from build123d import *

# Parameters (mm, degrees)
SKETCH3_R           = 57.15
BOSS_EXTRUDE2_DEPTH = 6.35
SKETCH4_R           = 3.81
SKETCH4_R_2         = 12.7
CUT_EXTRUDE1_DEPTH  = 6.35
SKETCH5_R           = 1.9685
CUT_EXTRUDE2_DEPTH  = 6.35


with BuildPart() as part:
    # Sketch3 → Boss-Extrude2 (new body)
    with BuildSketch(Plane.XY):
        Circle(SKETCH3_R)
    extrude(amount=BOSS_EXTRUDE2_DEPTH)

    # Sketch4 → Cut-Extrude1 (cut)
    with BuildSketch(Plane(origin=(0, 0, 0), x_dir=(-1, 0, 0), z_dir=(0, 0, -1))):
        with Locations((-35.921024484, 35.921024484)):
            Circle(SKETCH4_R)
        with Locations((35.921024484, 35.921024484)):
            Circle(SKETCH4_R)
        with Locations((35.921024484, -35.921024484)):
            Circle(SKETCH4_R)
        with Locations((-35.921024484, -35.921024484)):
            Circle(SKETCH4_R)
        Circle(SKETCH4_R_2)
    extrude(amount=-CUT_EXTRUDE1_DEPTH, mode=Mode.SUBTRACT)

    # Sketch5 → Cut-Extrude2 (cut)
    with BuildSketch(Plane.XY.offset(6.35)):
        with Locations((-22.225, 22.225)):
            Circle(SKETCH5_R)
        with Locations((22.225, 22.225)):
            Circle(SKETCH5_R)
        with Locations((22.225, -22.225)):
            Circle(SKETCH5_R)
        with Locations((-22.225, -22.225)):
            Circle(SKETCH5_R)
    extrude(amount=-CUT_EXTRUDE2_DEPTH, mode=Mode.SUBTRACT)


solid = part.part
The listing builds one solid part. Answer for the finished solid, in the listing's coordinates (mm). Coordinates: 2 decimals unless noted, no trailing zeros. Write each loop counter-clockwise with the first axis right and the second up, starting at its lowest first coordinate (ties: lowest second). Pieces come first, ordered by that corner, then holes. Notation, with made-up numbers: M -1,-40 L 43,-40 A30 cw 43,-3 Z; hole C 46.25,21.5 d2. An arc over 180 degrees is marked long. Write each question's results on one line, items separated by ' | '.
Item 1: Consider probe 1 along Y at (x, z) = (36, 2); probe 2 along Y at (x, z) = (-23, 5.75); probe 3 along Y at (x, z) = (0, 3.75). Determine where each line is inside the solid, lowest interval first. Write a range as [from, to].
Answer below:
probe 1: [-44.39, -39.73], [-32.11, 32.11], [39.73, 44.39] | probe 2: [-52.32, -24.03], [-20.42, 20.42], [24.03, 52.32] | probe 3: [-57.15, -12.7], [12.7, 57.15]
Item 2: The part is cut by section D-D on z = 1.75. State how many separate pieces and enclosed holes the cut face has, and give its area (3 significant figures).
Answer below:
separate pieces: 1 | enclosed holes: 9 | area: 9,520 mm2
Item 3: The part is cut by section A-A on y = 0. Determine the outline of the cut face in (x, z).
Answer below:
outline: M -57.15,0 L -12.7,0 L -12.7,6.35 L -57.15,6.35 Z; M 12.7,0 L 57.15,0 L 57.15,6.35 L 12.7,6.35 Z
Item 4: Given P1, Ø2, axis at y = -17, z = 2, coming from the -X side; P2, Ø4.5, axis at x = 35.92, y = 35.92, coming from the +Z side; P3, Ø3, axis at y = -30.5, z = 4, coming from the +X side; P4, Ø2, axis at x = -6, z = 2, coming from the -Y side, each flat-ended and moving along its own axis, determine where each tip first touches the part or whether it passes through.
Answer below:
P1: x = -54.86 | P2: through | P3: x = 49.25 | P4: y = -56.93
Item 5: For a pull along X with two mould halves and no side action, classify faces 1 (the face through (-14, 1, 0)), 2 (the face through (-57.095, 2.513, 3.131)), 3 (the face through (39.727, 36.089, 3.131)) as released by +X, released by -X, zero draft, split by the parting line, or undercut.
Answer below:
face 1: zero draft | face 2: split by the parting line | face 3: undercut
Item 6: The part is cut by section C-C on x = -38. Determine the outline of the cut face in (y, z).
Answer below:
outline: M -42.69,0 L -39.11,0 L -39.11,6.35 L -42.69,6.35 Z; M -32.73,0 L 32.73,0 L 32.73,6.35 L -32.73,6.35 Z; M 39.11,0 L 42.69,0 L 42.69,6.35 L 39.11,6.35 Z
